The model under review builds one solid part; all positions refer to its coordinate system, in mm. A direction names the side the tool comes from. Coordinates: 2 decimals unless noted, no trailing zeros. Loops run counter-clockwise (first coordinate to the right, second up) from the corner with the lowest first, then second, coordinate; pieces in that order, holes last. Notation, with made-up numbers: M 52.5,26 L 72.5,26 A12 ccw 72.5,44 Z; hole C 86,17 d7. An arc over 180 degrees is marked long. One line per item, written item: value.
Autodesk Inventor part; units mm, degrees
ref_plane "YZ Plane" through (0, 0, 0) normal (1, 0, 0) x (0, 1, 0)
ref_plane "XZ Plane" through (0, 0, 0) normal (0, 1, 0) x (-1, 0, 0)
ref_plane "XY Plane" through (0, 0, 0) normal (0, 0, 1) x (1, 0, 0)
sketch "Sketch1" plane through (0, 0, 0) normal (0, 0, 1) x (1, 0, 0)
  line L0 (-63.5, -10.25) -> (63.5, -10.25)
  line L1 (63.5, -10.25) -> (63.5, 10.25)
  line L2 (63.5, 10.25) -> (-63.5, 10.25)
  line L3 (-63.5, 10.25) -> (-63.5, -10.25)
  line L4 (-63.5, -10.25) -> (63.5, 10.25) construction
  line L5 (63.5, -10.25) -> (-63.5, 10.25) construction
  line L6 (-63.5, -5) -> (-60.5, -5)
  line L7 (-60.5, -5) -> (-60.5, 5) construction
  line L8 (-60.5, 5) -> (-63.5, 5)
  line L9 (-63.5, 5) -> (-63.5, -5)
  line L10 (-63.5, -5) -> (-60.5, 5) construction
  line L11 (-60.5, -5) -> (-63.5, 5) construction
  line L12 (-45, -10.25) -> (-25, -10.25)
  line L13 (-25, -10.25) -> (-25, -7.25)
  line L14 (-25, -7.25) -> (-45, -7.25) construction
  line L15 (-45, -7.25) -> (-45, -10.25)
  line L16 (-45, -10.25) -> (-25, -7.25) construction
  line L17 (-25, -10.25) -> (-45, -7.25) construction
  line L18 (-10, -10.25) -> (10, -10.25)
  line L19 (10, -10.25) -> (10, -7.25)
  line L20 (10, -7.25) -> (-10, -7.25) construction
  line L21 (-10, -7.25) -> (-10, -10.25)
  line L22 (-10, -10.25) -> (10, -7.25) construction
  line L23 (10, -10.25) -> (-10, -7.25) construction
  line L24 (25, -7.25) -> (25, -10.25)
  line L25 (45, -10.25) -> (45, -7.25)
  line L26 (25, -10.25) -> (45, -10.25)
  line L27 (45, -10.25) -> (25, -7.25) construction
  line L28 (45, -7.25) -> (25, -7.25) construction
  line L29 (25, -10.25) -> (45, -7.25) construction
  line L30 (-45, -7.25) -> (-63.5, -7.25)
  line L31 (-25, -7.25) -> (-10, -7.25)
  line L32 (10, -7.25) -> (25, -7.25)
  line L33 (45, -7.25) -> (63.5, -7.25)
  line L34 (-60.5, 5) -> (-60.5, 10.25)
  line L35 (-60.5, -5) -> (-60.5, -10.25)
  point P0 (0, 0)
  point P1 (-62, 0)
  point P2 (-63.5, 0)
  point P3 (-35, -8.75)
  point P4 (0, -8.75)
  point P5 (35, -8.75)
  point P6 (0, -10.25)
  point P7 (-45, -10.25)
  point P8 (-25, -10.25)
  point P9 (-10, -10.25)
  point P10 (10, -10.25)
  point P11 (25, -10.25)
  point P12 (45, -10.25)
  point P13 (-60.5, -7.25)
  dimension "d0" = 20.5
  dimension "d1" = 127
  dimension "d2" = 10
  dimension "d3" = 3
  dimension "d4" = 3
  dimension "d5" = 20
  dimension "d6" = 3
  dimension "d7" = 20
  dimension "d8" = 35
  dimension "d9" = 3
  dimension "d10" = 20
  dimension "d11" = 35
extrude "Extrusion1" add sketch "Sketch1" along normal blind 3 contours L3 L6 L35 L30 | L15 L30 L35 L6 L3 L8 L34 L2 L1 L33 L25 L0 L24 L32 L19 L21 L31 L13 | L3 L2 L34 L8
extrude "Extrusion2" cut sketch "Sketch1" along normal through all contours L3 L30 L35 L0 | L35 L30 L15 L0 | L3 L6 L35 L30 | L13 L31 L21 L0 | L3 L2 L34 L8 | L19 L32 L24 L0 | L25 L33 L1 L0
mirror "Mirror1" about plane through (0, 0, 0) normal (1, 0, 0) of "Extrusion2"
equation "\"d4\" = d3"
equation "\"d6\" = d3"
equation "\"d7\" = d5"
equation "\"d9\" = d6"
equation "\"d10\" = d7"
properties part number "bed_acrylic_upper_front"
(1) To check wall thickness, follow L1, parallel to X at y = -8, z = 1.4; L2, parallel to Y at x = -14, z = 2.6; L3, parallel to X at y = -6.75, z = 0.25. State the ranges of each line that lie inside material, in increasing order. Write a range as [from, to].
Checks:
L1: [-45, -25], [-10, 10], [25, 45]
L2: [-7.25, 10.25]
L3: [-60.5, 60.5]
(2) Add section C-C on x = -16.5. State the section outline as (y, z) points.
Checks:
outline: M -7.25,0 L 10.25,0 L 10.25,3 L -7.25,3 Z
(3) Draft analysis for pull direction X (two halves, no side actions). For faces 4 (the face through (-45, -9, 1)), 5 (the face through (-25, -9, 1)), 6 (the face through (1, 10.25, 1)), state which applies: pulls with the +X half, pulls with the -X half, needs draft (parallel to the pull), parting line crosses it, or undercut.
Checks:
face 4: pulls with the -X half
face 5: undercut
face 6: needs draft
(4) Add section A-A on z = 1.15. State the section outline as (x, y) points, then the cut area to 3 significant figures.
Checks:
outline: M -63.5,-5 L -60.5,-5 L -60.5,-7.25 L -45,-7.25 L -45,-10.25 L -25,-10.25 L -25,-7.25 L -10,-7.25 L -10,-10.25 L 10,-10.25 L 10,-7.25 L 25,-7.25 L 25,-10.25 L 45,-10.25 L 45,-7.25 L 60.5,-7.25 L 60.5,-5 L 63.5,-5 L 63.5,5 L 60.5,5 L 60.5,10.25 L -60.5,10.25 L -60.5,5 L -63.5,5 Z
area: 2,360 mm^2
(5) Tool access review of faces 1 (the face through (60.5, 8, 1)), 2 (the face through (-53, -7.25, 1)), 3 (the face through (25, -9, 1)): name each direction out of +Z, -Z, +X, -X, +Y, -Y from which nothing blocks a thin tool from reaching the whole face with its end or side.
Checks:
face 1: +Z, -Z, +X, +Y
face 2: +Z, -Z, -X, -Y
face 3: +Z, -Z, -Y
(6) Insertion check: pin 1 Ø1.5 at (x, z) = (54.5, 1) entering from -Y; pin 2 Ø0.7 at (y, z) = (-6, 1.5) entering from +X; pin 3 Ø0.9 at (y, z) = (-8, 1.5) entering from +X. Each pin has a flat end and moves straight along its axis. Give the tip position at first contact, or say it passes through.
Checks:
pin 1: y = -7.25
pin 2: x = 60.5
pin 3: x = 45
(7) Add section B-B on y = 7.25. State the section outline as (x, z) points, then the cut area to 3 significant figures.
Checks:
outline: M -60.5,0 L 60.5,0 L 60.5,3 L -60.5,3 Z
area: 363 mm^2
